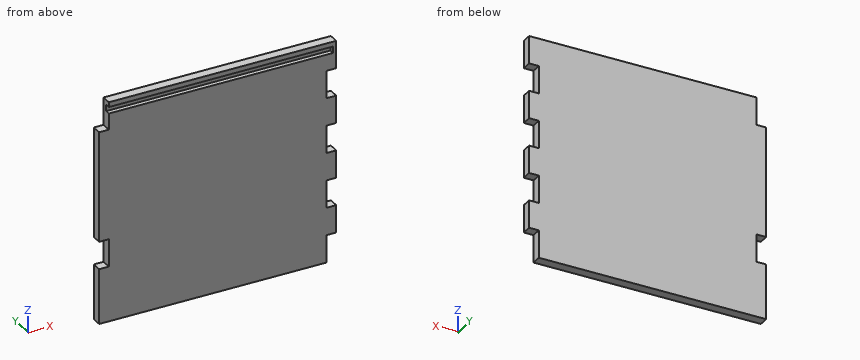
```python
from build123d import *

# Parameters (mm, degrees)
F1_DEPTH = 19.05
F2_W     = 9.525
F2_H     = 12.7
F3_DEPTH = 438.15


with BuildPart() as f1:
    # F0 (on Front) → F1 (new body)
    with BuildSketch(Plane.XZ):
        Polygon((0, 107.95), (0, 0), (444.5, 0), (444.5, 53.975), (463.55, 53.975), (463.55, 107.95), (444.5, 107.95), (444.5, 161.925), (463.55, 161.925), (463.55, 215.9), (444.5, 215.9), (444.5, 269.875), (463.55, 269.875), (463.55, 323.85), (444.5, 323.85), (444.5, 377.825), (463.55, 377.825), (463.55, 431.8), (19.05, 431.8), (19.05, 377.825), (0, 377.825), (0, 161.925), (19.05, 161.925), (19.05, 107.95), align=None)
    extrude(amount=F1_DEPTH)

    # F2 (on face) → F3 (cut)
    with BuildSketch(Plane(origin=(19.05, 0, 0), x_dir=(0, -1, 0), z_dir=(-1, 0, 0))):
        with Locations((14.2875, 415.925)):
            Rectangle(F2_W, F2_H)
    extrude(amount=-F3_DEPTH, mode=Mode.SUBTRACT)


solid = f1.part
```
The model under review builds one solid part; all positions refer to its coordinate system, in mm. Round coordinates to 2 decimals unless told otherwise and drop trailing zeros. Write each loop counter-clockwise with the first axis right and the second up, starting at its lowest first coordinate (ties: lowest second). Pieces come first, ordered by that corner, then holes. Notation, with made-up numbers: (-8, 50.25) - (22, 50.25) arc R26 cw to (22, 87.25) - close; hole circle Ø11 at (11, -1). An arc over 180 degrees is marked (long way). Answer as CSV lines item,"result". Start each with the question number.
(1) To check wall thickness, follow line 1 (Z direction, x = 439, y = -17.5) (3 decimals); line 2 (X direction, y = -4.25, z = 367); line 3 (X direction, y = -9, z = 378). State the ranges of each line that lie inside material, in increasing order.
(2) We need section A-A on y = -13. State the section outline as (x, z) points (3 decimals).
(3) We need section B-B on z = 230. State the section outline as (x, y) points, plus the area to 3 significant figures.
(4) For pin 1 Ø5 at (x, y) = (305.5, -16) entering from -Z; pin 2 Ø5 at (y, z) = (-15, 416) entering from -X; pin 3 Ø9.5 at (x, y) = (10.5, -13.5) entering from +Z (3 decimals); pin 4 Ø9.5 at (y, z) = (-13, 244.5) entering from +X, all flat-tipped, find the tip position at first contact; note any pin that passes through.
Worked answers:
1,line 1,"0 to 409.575, 422.275 to 431.8"
1,line 2,"0 to 444.5"
1,line 3,"19.05 to 463.55"
2,outline,"(0, 0) - (444.5, 0) - (444.5, 53.975) - (463.55, 53.975) - (463.55, 107.95) - (444.5, 107.95) - (444.5, 161.925) - (463.55, 161.925) - (463.55, 215.9) - (444.5, 215.9) - (444.5, 269.875) - (463.55, 269.875) - (463.55, 323.85) - (444.5, 323.85) - (444.5, 377.825) - (463.55, 377.825) - (463.55, 431.8) - (19.05, 431.8) - (19.05, 422.275) - (457.2, 422.275) - (457.2, 409.575) - (19.05, 409.575) - (19.05, 377.825) - (0, 377.825) - (0, 161.925) - (19.05, 161.925) - (19.05, 107.95) - (0, 107.95) - close"
3,outline,"(0, -19.05) - (444.5, -19.05) - (444.5, 0) - (0, 0) - close"
3,area,"8,470 mm²"
4,pin 1,"z = 0"
4,pin 2,"x = 457.2"
4,pin 3,"z = 377.825"
4,pin 4,"x = 444.5"
